```python
from build123d import *

# Parameters (mm, degrees)
SKETCH1_W           = 76.2
SKETCH1_H           = 50.8
BOSS_EXTRUDE1_DEPTH = 2.54
SKETCH2_R           = 5.715
SKETCH2_R_2         = 3.175
BOSS_EXTRUDE2_DEPTH = 76.2
SKETCH3_W           = 25.4
SKETCH3_H           = 25.4
CUT_EXTRUDE1_DEPTH  = 93.291521279


with BuildPart() as part:
    # Sketch1 → Boss-Extrude1 (new body)
    with BuildSketch(Plane.XY):
        with Locations((-38.1, 25.4)):
            Rectangle(SKETCH1_W, SKETCH1_H)
    extrude(amount=BOSS_EXTRUDE1_DEPTH)

    # Sketch2 → Boss-Extrude2 (add)
    with BuildSketch(Plane.ZY.offset(76.2)):
        with Locations((5.715, 0)):
            Circle(SKETCH2_R)
        with Locations((5.715, 0)):
            Circle(SKETCH2_R_2, mode=Mode.SUBTRACT)
    extrude(amount=-BOSS_EXTRUDE2_DEPTH)

    # Sketch3 → Cut-Extrude1 (cut, through all)
    with BuildSketch(Plane(origin=(0, 0, 0), x_dir=(-1, 0, 0), z_dir=(0, 0, -1))):
        with Locations((19.05, -2.54)):
            Rectangle(SKETCH3_W, SKETCH3_H)
        with Locations((57.15, -2.54)):
            Rectangle(SKETCH3_W, SKETCH3_H)
    extrude(amount=-CUT_EXTRUDE1_DEPTH, mode=Mode.SUBTRACT)


solid = part.part
```
Source: CAD feature listing. Evaluate the final solid. Frame: model axes, mm. A direction names the side the tool comes from. Give positions to 0.01 mm unless a question says otherwise; leave off trailing zeros. Order: outer loops, then holes, each group sorted by start corner. A loop starts at its lowest first (then second) coordinate and runs counter-clockwise, first axis right, second up.
(1) Material intervals for line 1 along X through (y, z) = (4, 8.75); line 2 along Z through (x, y) = (-74, 0); line 3 along Y through (x, z) = (-53, 2), sorted ascending.
(2) Access query for faces 1 (the face through (-6.35, 2, 3)), 2 (the face through (-3.219, -1.932, 3.195)). Directions: +Z, -Z, +X, -X, +Y, -Y. A direction counts if a zero-diameter tool reaches every point of the face in a straight line with its end or side. Return the directions, or none.
(3) Section query D-D (y = 21.5). Return the cut outline in (x, z).
(4) Contact query for flat-ended pins moving along their axis: P1, Ø3.5, axis at y = 2, z = 8, coming from the -X side; P2, Ø5, axis at y = 0, z = 5.715, coming from the +X side; P3, Ø6, axis at x = -31, y = 44.5, coming from the +Z side; P4, Ø0.8, axis at x = -17.5, z = 1, coming from the -Y side. Output: stop coordinate, or through.
(5) Section query A-A (x = -37). Return the cut outline in (y, z) (3 decimals), plus the area to 3 significant figures.
(6) Section query C-C (z = 4). Return the cut outline in (x, y).
(7) Section query B-B (z = 8). Return the cut outline in (x, y).
(8) Pull-direction query (X, two-part tool) for faces 3 (the face through (-69.85, 2, 3)), 4 (the face through (0, 16, 2)), 5 (the face through (-73.069, -1.932, 3.195)); classes: +X half, -X half, draft (parallel to the pull), parting line (faces both ways), or undercut.
Outcome:
1. line 1: x = -76.2 to -69.85, -44.45 to -31.75, -6.35 to 0
1. line 2: z = 0 to 2.54, 8.89 to 11.43
1. line 3: y = 10.16 to 50.8
2. face 1: +Z, -Z, -Y
2. face 2: +X, -X
3. outline: (-76.2, 0) - (0, 0) - (0, 2.54) - (-76.2, 2.54) - close
4. P1: stops at x = -76.2
4. P2: passes through
4. P3: stops at z = 2.54
4. P4: stops at y = 10.16
5. outline: (0, 0) - (50.8, 0) - (50.8, 2.54) - (4.752, 2.54) arc R5.715 ccw (long way) to start; hole circle Ø6.35 at (0, 5.715)
5. area: 191 mm2
6. outline: (-76.2, -5.45) - (-69.85, -5.45) - (-69.85, -2.67) - (-76.2, -2.67) - close; (-76.2, 2.67) - (-69.85, 2.67) - (-69.85, 5.45) - (-76.2, 5.45) - close; (-44.45, -5.45) - (-31.75, -5.45) - (-31.75, -2.67) - (-44.45, -2.67) - close; (-44.45, 2.67) - (-31.75, 2.67) - (-31.75, 5.45) - (-44.45, 5.45) - close; (-6.35, -5.45) - (0, -5.45) - (0, -2.67) - (-6.35, -2.67) - close; (-6.35, 2.67) - (0, 2.67) - (0, 5.45) - (-6.35, 5.45) - close
7. outline: (-76.2, -5.24) - (-69.85, -5.24) - (-69.85, -2.2) - (-76.2, -2.2) - close; (-76.2, 2.2) - (-69.85, 2.2) - (-69.85, 5.24) - (-76.2, 5.24) - close; (-44.45, -5.24) - (-31.75, -5.24) - (-31.75, -2.2) - (-44.45, -2.2) - close; (-44.45, 2.2) - (-31.75, 2.2) - (-31.75, 5.24) - (-44.45, 5.24) - close; (-6.35, -5.24) - (0, -5.24) - (0, -2.2) - (-6.35, -2.2) - close; (-6.35, 2.2) - (0, 2.2) - (0, 5.24) - (-6.35, 5.24) - close
8. face 3: undercut
8. face 4: +X half
8. face 5: draft
